Work out the finished part from the listing and answer in its coordinate system (mm). A direction names the side the tool comes from. Coordinates: 2 decimals unless noted, no trailing zeros. Order: outer loops, then holes, each group sorted by start corner. A loop starts at its lowest first (then second) coordinate and runs counter-clockwise, first axis right, second up. Notation, with made-up numbers: M 32.25,12.25 L 82.25,12.25 A23 cw 82.25,45.25 Z; hole C -24.75,-10.5 d9. An arc over 180 degrees is marked long. Write item = value, one per line. Start each with the question number.
Q1. Find section C-C on y = 450. Give the vertices of the cut face in (x, z).
Q2. Find section B-B on z = -142. Give the vertices of the cut face in (x, y), and give its area (3 significant figures).
Q3. Each of these flat-tipped pins is pushed along its axis until it touches: P1, Ø12, axis at y = 255, z = -37, coming from the +X side; P2, Ø10, axis at y = 268, z = -210.5, coming from the -X side; P3, Ø6, axis at y = 536.5, z = -684, coming from the +X side. Where does it stop, or does it pass through?
Q4. A tool of negligible diameter and unlimited length cuts with its end or side. For faces 5 (the cylindrical face through (358.637, 559.428, -728.893)), 6 (the cylindrical face through (-332.082, 559.428, -728.893)), 7 (the flat face through (-655.725, 565, -699)), from which of +Z, -Z, +X, -X, +Y, -Y can it reach the whole face along a straight path? Write none if from no direction.
Q5. Find section A-A on y = 636.5. Give the vertices of the cut face in (x, z).
Q6. Find section D-D on z = -14. Give the vertices of the cut face in (x, y).
Q7. Straight lines are drawn through the part: line 1 along X through (y, z) = (384.5, -434.5); line 2 along X through (y, z) = (447, -460); line 3 along Z through (x, y) = (577, 578.5). For each, find the intervals that lie inside material, in ascending order.
Q8. Determine the mould class of faces 1 (the cylindrical face through (46.376, 235.346, -140.421)), 2 (the flat face through (1, 762, -761)), 3 (the flat face through (17.375, 342, -357)), 4 (the cylindrical face through (-1.1, 328.6, -45.1)) for opening direction Z: released by +Z, released by -Z, zero draft, split by the parting line, or undercut.
```python
from build123d import *

# Parameters (mm, degrees)
F3_R     = 29.6946462183
F4_DEPTH = 673.1
F5_R     = 31.777125294
F5_R_2   = 32.6810684337
F6_DEPTH = 673.101


# Not quite as in the source:
# - a feature of the source that left no trace in its solid (it failed there, or was rolled back) is left out


with BuildPart() as f2:
    # F2: sweep along a path in F1
    with BuildLine(Plane.YZ) as f2_path:
        ThreePointArc((0, 0), (269.4076836321, -111.5923163679), (381, -381))
        ThreePointArc((381, -381), (492.5923163679, -650.4076836321), (762, -762))
    # F0 (on Front) → F2 (sweep)
    with BuildSketch(Plane.XZ):
        Polygon((76.2, 88.9), (0, 88.9), (-76.2, 88.9), (-76.2, 44.45), (-17.3748321831, 44.45), (-17.3748321831, 0), (-17.3748321831, -44.45), (-76.2, -44.45), (-76.2, -88.9), (0, -88.9), (76.2, -88.9), (76.2, -44.45), (17.3748321831, -44.45), (17.3748321831, 0), (17.3748321831, 44.45), (76.2, 44.45), align=None)
    sweep(path=f2_path.line)

    # F3 (on face) → F4 (join, symmetric)
    with BuildSketch(Plane.YZ.offset(17.3748321831)):
        with Locations((565.865278244, -699.9046206474)):
            Circle(F3_R)
    extrude(amount=F4_DEPTH, both=True)

    # F5 (on face) → F6 (cut, through all)
    with BuildSketch(Plane.YZ.offset(17.3748321831)):
        with Locations((631.9480538368, -732.2566509247)):
            Circle(F5_R)
        with Locations((709.6602916718, -753.0537247658)):
            Circle(F5_R_2)
    extrude(amount=-F6_DEPTH, mode=Mode.SUBTRACT)


solid = f2.part
```
Findings below:
q1.outline = M -76.2,-732.37 L 76.2,-732.37 L 76.2,-670.25 L 17.37,-670.25 L 17.37,-507.18 L 76.2,-507.18 L 76.2,-245.7 L -76.2,-245.7 L -76.2,-507.18 L -17.37,-507.18 L -17.37,-670.25 L -76.2,-670.25 Z
q2.outline = M -76.2,167.93 L 76.2,167.93 L 76.2,236.95 L 17.37,236.95 L 17.37,351.98 L 76.2,351.98 L 76.2,404.58 L -76.2,404.58 L -76.2,351.98 L -17.37,351.98 L -17.37,236.95 L -76.2,236.95 Z
q2.area = 22,500 mm^2
q3.P1 = 76.2
q3.P2 = -76.2
q3.P3 = 17.37
q4.face_5 = +X
q4.face_6 = -X
q4.face_7 = +Z, -Z, -X, +Y, -Y
q5.outline = M -76.2,-833.83 L 76.2,-833.83 L 76.2,-787.52 L 17.37,-787.52 L 17.37,-763.71 L -17.37,-763.71 L -17.37,-787.52 L -76.2,-787.52 Z; M -76.2,-693.27 L -17.37,-693.27 L -17.37,-700.81 L 17.37,-700.81 L 17.37,-693.27 L 76.2,-693.27 L 76.2,-644.77 L -76.2,-644.77 Z
q6.outline = M -76.2,215.22 L -17.37,215.22 L -17.37,0 L 17.37,0 L 17.37,215.22 L 76.2,215.22 L 76.2,293.46 L -76.2,293.46 Z
q7.line_1 = -17.37 to 17.37
q7.line_2 = -76.2 to 76.2
q7.line_3 = -726.78 to -673.03
q8.face_1 = undercut
q8.face_2 = zero draft
q8.face_3 = undercut
q8.face_4 = released by +Z
